Model file for the job. Use its own axes, mm. Face numbers are marked on the shaded views. Coordinates: 2 decimals unless noted, no trailing zeros. Loops run counter-clockwise (first coordinate to the right, second up) from the corner with the lowest first, then second, coordinate; pieces in that order, holes last.
Autodesk Inventor part; units mm, degrees
ref_plane "YZ Plane" through (0, 0, 0) normal (1, 0, 0) x (0, 1, 0)
ref_plane "XZ Plane" through (0, 0, 0) normal (0, 1, 0) x (-1, 0, 0)
ref_plane "XY Plane" through (0, 0, 0) normal (0, 0, 1) x (1, 0, 0)
sketch "Sketch1" plane through (0, 0, 0) normal (0, 1, 0) x (-1, 0, 0)
  line L0 (0, 0) -> (2.5, 0)
  line L1 (2.5, -1.4434) -> (0, -2.8868)
  line L2 (0, -2.8868) -> (-2.5, -1.4434)
  line L3 (-2.5, -1.4434) -> (-2.5, 1.4434)
  line L4 (-2.5, 1.4434) -> (0, 2.8868)
  line L5 (0, 2.8868) -> (2.5, 1.4434)
  line L6 (2.5, 1.4434) -> (2.5, -1.4434)
  dimension "d0" = 2.5
extrude "Extrusion1" add sketch "Sketch1" along normal blind 15
sketch "Sketch2" plane through (0, 15, 0) normal (0, 1, 0) x (1, 0, 0)
  point P0 (0, 0)
hole "Hole1" at (0, 15, 0) direction (0, -1, 0) diameter 2.459 end through all
chamfer "Chamfer1" distance 0.5 angle 45 2 edges at (0, 15, -1.2295) (0, 0, -1.2295)
properties part number "18mm Standoff" material "Aluminum 6061"
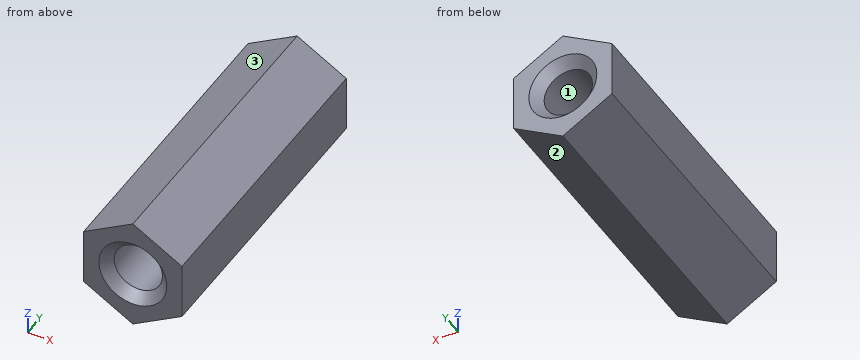
Q1. Mould opens along Z. For the marked faces 1, 2 and 3 say: +Z half, -Z half, draft (parallel to the pull), parting line (faces both ways), or undercut.
Answers:
face 1: undercut
face 2: -Z half
face 3: +Z half
Q2. Slice it at B-B (y = 14.25). List the corners of the cut face in (x, z), and give its area (3 significant figures).
Answers:
outline: (-2.5, -1.44) - (0, -2.89) - (2.5, -1.44) - (2.5, 1.44) - (0, 2.89) - (-2.5, 1.44) - close; hole circle Ø2.46 at (0, 0)
area: 16.9 mm2
Q3. Slice it at A-A (z = 0). List the corners of the cut face in (x, y).
Answers:
outline: (-2.5, 0) - (-1.73, 0) - (-1.23, 0.5) - (-1.23, 14.5) - (-1.73, 15) - (-2.5, 15) - close; (1.23, 0.5) - (1.73, 0) - (2.5, 0) - (2.5, 15) - (1.73, 15) - (1.23, 14.5) - close
Q4. Drill centre lines: line 1 (X direction, y = 4, z = 0); line 2 (X direction, y = 3, z = -0.65); line 3 (Z direction, x = 0.5, y = 3.5). Where is each one in solid material? Low to high.
Answers:
line 1: x = -2.5 to -1.23, 1.23 to 2.5
line 2: x = -2.5 to -1.04, 1.04 to 2.5
line 3: z = -2.6 to -1.12, 1.12 to 2.6
Q5. Flat gauge pins, fed straight in: P1, Ø2, axis at x = -1.5, z = 0.5, coming from the -Y side; P2, Ø2, axis at x = 2, y = 5.5, coming from the +Z side. Where does each tip first touch, or does it go through?
Answers:
P1: stops at y = 0
P2: stops at z = 2.31
